Can you work these out from the model? Positions are in its coordinate system, mm. Coordinates: 2 decimals unless noted, no trailing zeros. Write each loop counter-clockwise with the first axis right and the second up, starting at its lowest first coordinate (ties: lowest second). Pieces come first, ordered by that corner, then holes. Notation, with made-up numbers: (81.5, 26.25) - (106.5, 26.25) arc R19 cw to (106.5, 42.25) - close; hole circle Ø6 at (89.5, 52). An arc over 180 degrees is marked (long way). One line per question, with ' | ' between items. Start each with the question number.
from build123d import *

# Parameters (mm, degrees)
BOSS_EXTRUDE1_DEPTH = 200
SKETCH4_W           = 200
SKETCH4_H           = 1000
BOSS_EXTRUDE2_DEPTH = 60


with BuildPart() as part:
    # Sketch3 → Boss-Extrude1 (new body)
    with BuildSketch(Plane.ZY.offset(1220)):
        Polygon((0, 500), (75, 125), (75, -125), (0, -500), align=None)
    extrude(amount=-BOSS_EXTRUDE1_DEPTH)

    # Sketch4 → Boss-Extrude2 (add)
    with BuildSketch(Plane(origin=(0, 0, 0), x_dir=(-1, 0, 0), z_dir=(0, 0, -1))):
        with Locations((1120, 0)):
            Rectangle(SKETCH4_W, SKETCH4_H)
    extrude(amount=BOSS_EXTRUDE2_DEPTH)


solid = part.part
(1) If we section it at B-B on z = 10: List the corners of the cut face in (x, y) for me, plus the area to 3 significant figures.
(2) If I drill on probe 1 along Z at (x, y) = (-1033, -293.5); probe 2 along Z at (x, y) = (-1042, 155.5), over which ranges is the centre line in solid material (lowest first)?
(3) If we section it at C-C on y = 300: List the corners of the cut face in (x, z) for me.
(4) I'm going to push flat-ended pins straight in: pin 1 (2 mm diameter, centred on x = -1134.5, y = 210.5, fed in from +Z); pin 2 (5 mm diameter, centred on x = -1175.5, y = 260, fed in from +Z). Where does each tip first touch, or does it pass through?
(5) If we section it at A-A on x = -1062: List the corners of the cut face in (y, z) for me.
Values:
1) outline: (-1220, -450) - (-1020, -450) - (-1020, 450) - (-1220, 450) - close | area: 180,000 mm2
2) probe 1: -60 to 41.3 | probe 2: -60 to 68.9
3) outline: (-1220, -60) - (-1020, -60) - (-1020, 40) - (-1220, 40) - close
4) pin 1: z = 58.1 | pin 2: z = 48.5
5) outline: (-500, -60) - (500, -60) - (500, 0) - (125, 75) - (-125, 75) - (-500, 0) - close
